```python
from build123d import *

# Parameters (mm, degrees)
F0_W     = 762
F0_H     = 590.55
F1_DEPTH = 19.05
F3_DEPTH = 25.4
F5_DEPTH = 25.4
F7_DEPTH = 25.4
F9_DEPTH = 25.4


with BuildPart() as f1:
    # F0 (on Top) → F1 (new body)
    with BuildSketch(Plane.XY):
        Rectangle(F0_W, F0_H)
    extrude(amount=F1_DEPTH)

    # F2 (on face) → F3 (cut)
    with BuildSketch(Plane.XY.offset(19.05)):
        with BuildLine():
            ThreePointArc((-381, -142.875), (-224.904359, 52.476061), (-165.1, 295.275))
            Line((-165.1, 295.275), (-381, 295.275))
            Line((-381, 295.275), (-381, -142.875))
        make_face()
    extrude(amount=-F3_DEPTH, mode=Mode.SUBTRACT)

    # F4 (on face) → F5 (cut)
    with BuildSketch(Plane.XY.offset(19.05)):
        with BuildLine():
            Line((381, 22.225), (381, 295.275))
            Line((381, 295.275), (273.05, 295.275))
            ThreePointArc((273.05, 295.275), (306.438019, 150.610961), (381, 22.225))
        make_face()
    extrude(amount=-F5_DEPTH, mode=Mode.SUBTRACT)

    # F6 (on face) → F7 (cut)
    with BuildSketch(Plane.XY.offset(19.05)):
        Polygon((381, -295.275), (381, 22.225), (330.2, -295.275), align=None)
    extrude(amount=-F7_DEPTH, mode=Mode.SUBTRACT)

    # F8 (on face) → F9 (cut)
    with BuildSketch(Plane.XY.offset(19.05)):
        Polygon((-349.161536, -233.895749), (-381, -142.875), (-381, -295.275), (-270.685613, -295.275), align=None)
    extrude(amount=-F9_DEPTH, mode=Mode.SUBTRACT)


solid = f1.part
```
Geometry: final body of the model. Coordinates: model frame, mm. Give positions to 0.01 mm unless a question says otherwise; leave off trailing zeros. Loops run counter-clockwise (first coordinate to the right, second up) from the corner with the lowest first, then second, coordinate; pieces in that order, holes last. Notation, with made-up numbers: (83, -6) - (106, -6) arc R11 cw to (106, 1) - close; hole circle Ø9 at (50.25, 69). An arc over 180 degrees is marked (long way). Answer as CSV lines item,"result". Start each with the question number.
(1) Section query A-A (z = 14.75). Output: boundary loops of the cut face in (x, y) (3 decimals).
(2) Ray query, line 1 along X through (y, z) = (69, 5); line 2 along X through (y, z) = (22, 11.5); line 3 along Y through (x, z) = (-336.5, 12.5). Return the intervals inside material, ascending. Write a range as [from, to].
(3) Section query C-C (y = 196.5). Output: boundary loops of the cut face in (x, z), and give its area (3 significant figures).
(4) Section query B-B (x = 298). Output: boundary loops of the cut face in (y, z) (3 decimals).
(5) Pin query (flat end, axial travel): P1, Ø1, axis at x = -256.5, y = -216.5, coming from the -Z side. Return the tip coordinate at first contact, or that it passes through.
Worked answers:
1,outline,"(-381, -142.875) - (-349.162, -233.896) - (-270.686, -295.275) - (330.2, -295.275) - (381, 22.225) arc R497.854 cw to (273.05, 295.275) - (-165.1, 295.275) arc R582.485 cw to start"
2,line 1,"x = [-217.08, 347.74]"
2,line 2,"x = [-241.06, 380.96]"
2,line 3,"y = [-243.8, -102.92]"
3,outline,"(-176.07, 0) - (290.83, 0) - (290.83, 19.05) - (-176.07, 19.05) - close"
3,area,"8,890 mm^2"
4,outline,"(-295.275, 0) - (173.591, 0) - (173.591, 19.05) - (-295.275, 19.05) - close"
5,P1,"stops at z = 0"
